Input: dimensioned drawing with shaded views. Units: mm. Origin: part minimum x, y, z. Round coordinates to 2 decimals unless told otherwise and drop trailing zeros. Order: outer loops, then holes, each group sorted by start corner. A loop starts at its lowest first (then second) coordinate and runs counter-clockwise, first axis right, second up. Notation, with made-up numbers: M 77,27 L 129,27 A13 cw 129,36 Z; hole C 78.5,67 d5. An arc over 180 degrees is marked long. Use one line per item in the form item = value. Start each with the question number.
Q1. Section A-A (y = 1.3). Return the cut outline in (x, z) (3 decimals).
Q2. Section C-C (z = 2.5). Return the cut outline in (x, y) (3 decimals), plus the area to 3 significant figures.
Q3. Pull-direction query (Z, two-part tool) for the marked faces 1 and 2; classes: pulls with the +Z half, pulls with the -Z half, needs draft (parallel to the pull), parting line crosses it, or undercut.
Q4. Material intervals for probe 1 along Z at (x, y) = (19, 1.05) (1 decimal); probe 2 along Z at (x, y) = (85, 2.25) (3 decimals); probe 3 along X at (y, z) = (2, 9) (3 decimals), sorted ascending.
Q5. Section D-D (x = 69.85). Return the cut outline in (y, z) (3 decimals).
Q6. Contact query for a flat-ended pin moving along its axis: pin 1 (5 mm diameter, centred on x = 12.5, z = 6.5, fed in from -Y). Output: stop coordinate, or through.
Q7. Section B-B (x = 15). Return the cut outline in (y, z) (3 decimals), plus the area to 3 significant figures.
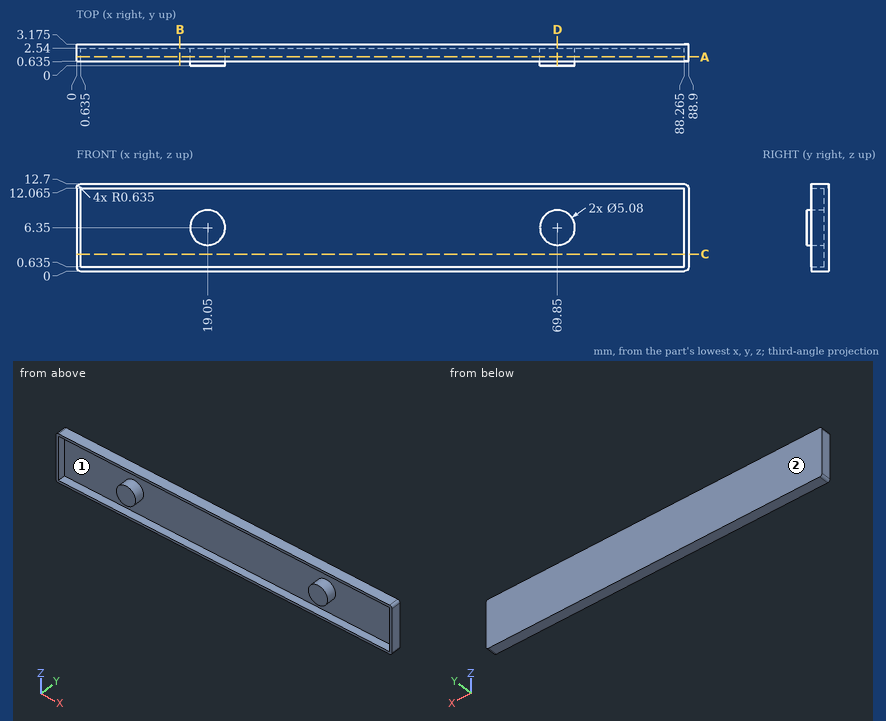
Results list:
q1.outline = M 0,0.635 A0.635 ccw 0.635,0 L 88.265,0 A0.635 ccw 88.9,0.635 L 88.9,12.065 A0.635 ccw 88.265,12.7 L 0.635,12.7 A0.635 ccw 0,12.065 Z; C 19.05,6.35 d5.08; C 69.85,6.35 d5.08; hole M 0.635,0.635 L 88.265,0.635 L 88.265,12.065 L 0.635,12.065 Z
q2.outline = M 0,0.635 L 0.635,0.635 L 0.635,2.54 L 88.265,2.54 L 88.265,0.635 L 88.9,0.635 L 88.9,3.175 L 0,3.175 Z
q2.area = 58.9 mm2
q3.face_1 = undercut
q3.face_2 = needs draft
q4.probe_1 = 0 to 0.6, 3.8 to 8.9, 12.1 to 12.7
q4.probe_2 = 0 to 0.635, 12.065 to 12.7
q4.probe_3 = 0 to 0.635, 88.265 to 88.9
q5.outline = M 0,3.81 L 2.54,3.81 L 2.54,0.635 L 0.635,0.635 L 0.635,0 L 3.175,0 L 3.175,12.7 L 0.635,12.7 L 0.635,12.065 L 2.54,12.065 L 2.54,8.89 L 0,8.89 Z
q6.pin_1 = 2.54
q7.outline = M 0.635,0 L 3.175,0 L 3.175,12.7 L 0.635,12.7 L 0.635,12.065 L 2.54,12.065 L 2.54,0.635 L 0.635,0.635 Z
q7.area = 10.5 mm2
